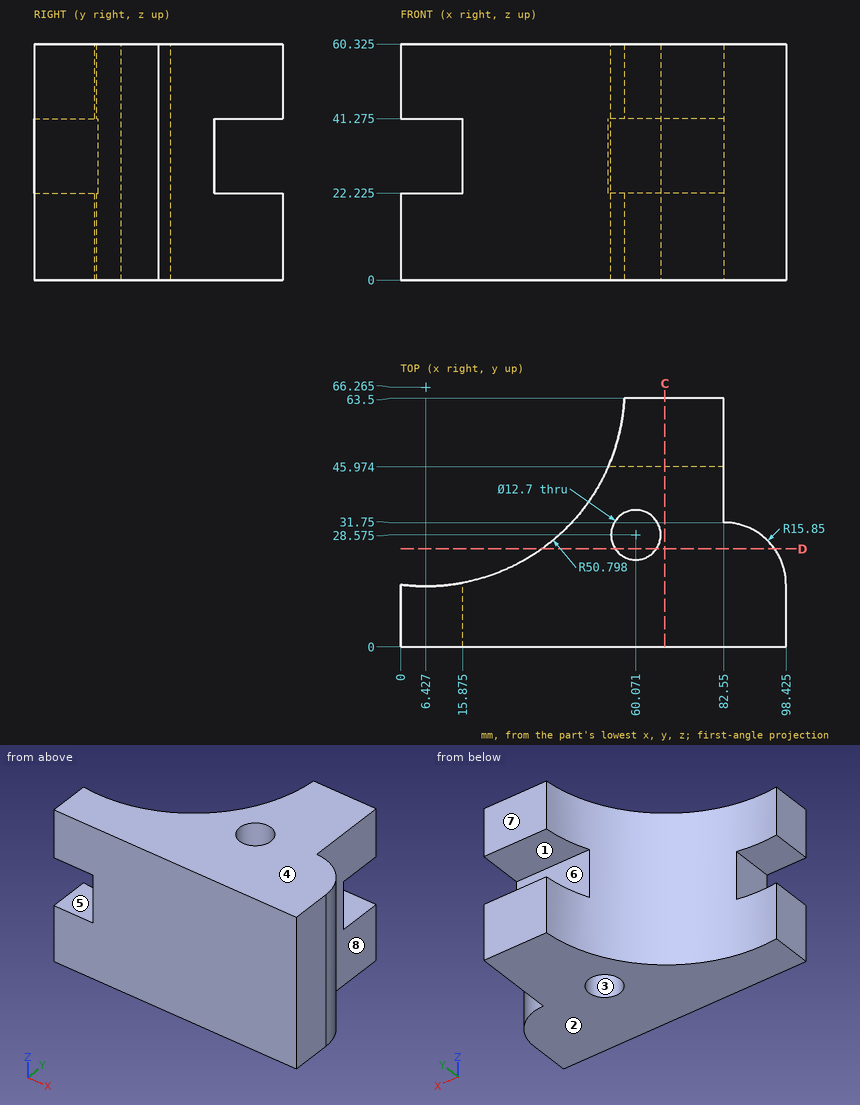
The drawing under review shows one solid part. Ordinate dimensions are in mm from its lowest x, y, z. A direction names the side the tool comes from. Round coordinates to 2 decimals unless told otherwise and drop trailing zeros. Order: outer loops, then holes, each group sorted by start corner. A loop starts at its lowest first (then second) coordinate and runs counter-clockwise, first axis right, second up. Notation, with made-up numbers: (-21.5, -39) - (13.5, -39) arc R32 cw to (13.5, -3) - close; hole circle Ø6 at (3, -2). An arc over 180 degrees is marked (long way). Return JSON: item names as keys, results as strings.
Q1. Machinability: for the marked faces 5, 6, 7 and 8, which of the approach directions +Z, -Z, +X, -X, +Y, -Y give a long, thin tool a straight path to every point of the face, cutting with its end or side? Answer none if there is none.
Computed values:
{"face 5": "-X, +Y, -Y", "face 6": "+X, -X, +Y", "face 7": "+Z, -Z, +X, -X, +Y", "face 8": "+Z, -Z, +X, +Y"}
Q2. For pin 1 Ø5.5 at (x, z) = (71, 29) entering from +Y; pin 2 Ø1.5 at (x, z) = (87.5, 27) entering from +Y; pin 3 Ø13 at (y, z) = (5, 32) entering from -X (3 decimals), all flat-tipped, find the tip position at first contact; note any pin that passes through.
Computed values:
{"pin 1": "stops at y = 45.97", "pin 2": "stops at y = 31.19", "pin 3": "stops at x = 15.875"}
Q3. The part is to be moulded in two halves that separate along Z. For the marked faces 1, 2, 3 and 4, say which applies: pulls with the +Z half, pulls with the -Z half, needs draft (parallel to the pull), parting line crosses it, or undercut.
Computed values:
{"face 1": "undercut", "face 2": "pulls with the -Z half", "face 3": "needs draft", "face 4": "pulls with the +Z half"}
Q4. Consider section C-C on x = 67.5. Write out the cut boundary in (y, z) (1 decimal).
Computed values:
{"outline": "(0, 0) - (63.5, 0) - (63.5, 22.2) - (46, 22.2) - (46, 41.3) - (63.5, 41.3) - (63.5, 60.3) - (0, 60.3) - close"}
Q5. Wall thickness on L1, parallel to Y at x = 59.5, z = 10; L2, parallel to Z at x = 76, y = 51.5 (1 decimal); L3, parallel to Y at x = 57.5, z = 13.5: over which ranges is each line inside the solid? List them lowest first. Write a range as [from, to].
Computed values:
{"L1": "y = [0, 22.25], [34.9, 63.5]", "L2": "z = [0, 22.2], [41.3, 60.3]", "L3": "y = [0, 22.77], [34.38, 63.5]"}
Q6. Consider section D-D on y = 25. Write out the cut boundary in (x, z) (1 decimal), plus the area to 3 significant figures.
Computed values:
{"outline": "(36.1, 0) - (54.8, 0) - (54.8, 60.3) - (36.1, 60.3) - close; (65.3, 0) - (95.6, 0) - (95.6, 60.3) - (65.3, 60.3) - close", "area": "2,960 mm2"}
